```python
from build123d import *

# Parameters (mm, degrees)
F0_R     = 30
F0_R_2   = 3
F1_DEPTH = 8
F2_T     = -7


with BuildPart() as f1:
    # F0 (on Top) → F1 (new body)
    with BuildSketch(Plane.XY):
        Circle(F0_R)
        with Locations((0, 20)):
            Circle(F0_R_2, mode=Mode.SUBTRACT)
    extrude(amount=F1_DEPTH)

    # F2
    f2_openings = [f1.faces().sort_by_distance(p)[0] for p in [
        (0, -0.20202, 8),
    ]]
    offset(amount=F2_T, openings=f2_openings)


solid = f1.part
```
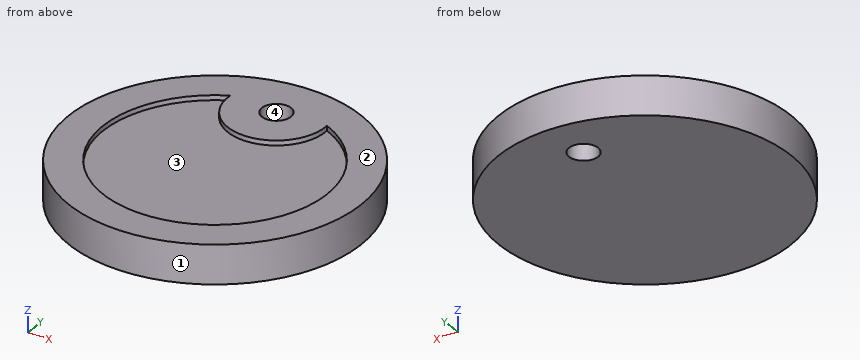
The listing builds one solid part. Answer for the finished solid, in the listing's coordinates (mm). Face numbers are marked on the shaded views. Round coordinates to 2 decimals unless told otherwise and drop trailing zeros. Loops run counter-clockwise (first coordinate to the right, second up) from the corner with the lowest first, then second, coordinate; pieces in that order, holes last.
1) A cutting plane is placed at A-A on x = 0. Determine the outline of the cut face in (y, z), plus the area to 3 significant figures.
Outcome:
outline: (-30, 0) - (17, 0) - (17, 8) - (10, 8) - (10, 7) - (-23, 7) - (-23, 8) - (-30, 8) - close; (23, 0) - (30, 0) - (30, 8) - (23, 8) - close
area: 399 mm2
2) A cutting plane is placed at C-C on z = 2. Determine the outline of the cut face in (x, y), plus the area to 3 significant figures.
Outcome:
outline: circle Ø60 at (0, 0); hole circle Ø6 at (0, 20)
area: 2,800 mm2
3) Given P1, Ø2, axis at y = -22, z = 4.5, coming from the +X side; P2, Ø1.5, axis at x = -4.5, z = 6.5, coming from the +Y side; P3, Ø1, axis at x = 9, z = 1.5, coming from the -Y side, each flat-ended and moving along its own axis, determine where each tip first touches the part or whether it passes through.
Outcome:
P1: stops at x = 21.42
P2: stops at y = 29.76
P3: stops at y = -28.77
4) A cutting plane is placed at B-B on y = 20. Determine the outline of the cut face in (x, z), plus the area to 3 significant figures.
Outcome:
outline: (-22.36, 0) - (-3, 0) - (-3, 8) - (-10, 8) - (-10, 7) - (-11.36, 7) - (-11.36, 8) - (-22.36, 8) - close; (3, 0) - (22.36, 0) - (22.36, 8) - (11.36, 8) - (11.36, 7) - (10, 7) - (10, 8) - (3, 8) - close
area: 307 mm2
5) A cutting plane is placed at D-D on y = 0. Determine the outline of the cut face in (x, z).
Outcome:
outline: (-30, 0) - (30, 0) - (30, 8) - (23, 8) - (23, 7) - (-23, 7) - (-23, 8) - (-30, 8) - close
6) Consider line 1 (Y direction, x = 0, z = 7.85); line 2 (Y direction, x = 0, z = 3.75); line 3 (Z direction, x = -5, y = -21.5). Determine where each line is inside the solid, lowest interval first.
Outcome:
line 1: y = -30 to -23, 10 to 17, 23 to 30
line 2: y = -30 to 17, 23 to 30
line 3: z = 0 to 7
7) For a pull along Y with two mould halves and no side action, classify the marked faces 1, 2, 3 and 4 as released by +Y, released by -Y, zero draft, split by the parting line, or undercut.
Outcome:
face 1: split by the parting line
face 2: zero draft
face 3: undercut
face 4: undercut
